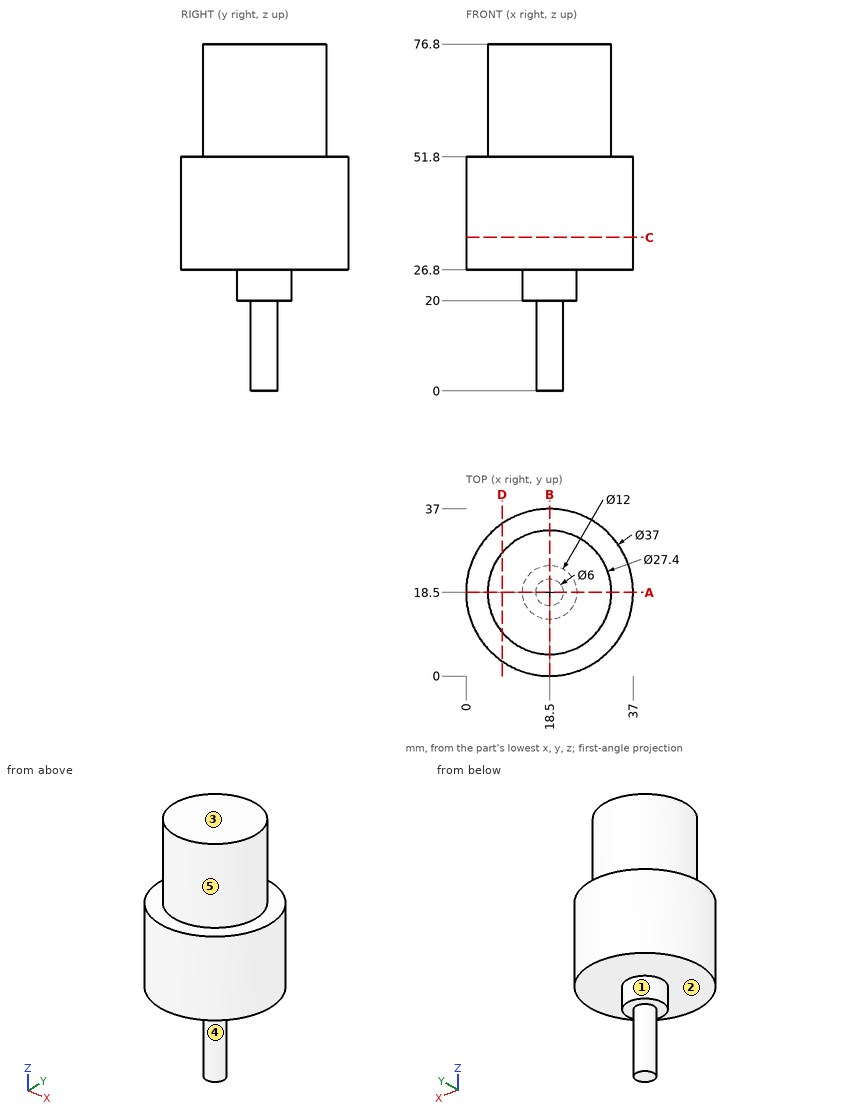
Source: three-view drawing plus pictorial views. Frame: mm from the lowest corner of the part. A direction names the side the tool comes from. Coordinates: 2 decimals unless noted, no trailing zeros. Write each loop counter-clockwise with the first axis right and the second up, starting at its lowest first coordinate (ties: lowest second). Pieces come first, ordered by that corner, then holes. Notation, with made-up numbers: (-3, 73.5) - (41, 73.5) arc R35 cw to (41, 108.5) - close; hole circle Ø6 at (-32, 30). An arc over 180 degrees is marked (long way). Answer as a JSON object with one key per item and string values.
Q1. Material intervals for line 1 (Z direction, x = 20, y = 25); line 2 (Z direction, x = 2, y = 15); line 3 (X direction, y = 29, z = 48), sorted ascending. Write a range as [from, to].
Ans:
{"line 1": "z = [26.8, 76.8]", "line 2": "z = [26.8, 51.8]", "line 3": "x = [3.27, 33.73]"}
Q2. Section query D-D, the plane x = 8. Output: boundary loops of the cut face in (y, z).
Ans:
{"outline": "(3.27, 26.8) - (33.73, 26.8) - (33.73, 51.8) - (27.3, 51.8) - (27.3, 76.8) - (9.7, 76.8) - (9.7, 51.8) - (3.27, 51.8) - close"}
Q3. First-contact query: pin 1 Ø12 at (x, z) = (26, 46.5) entering from +Y; pin 2 Ø6 at (x, z) = (21, 61.5) entering from +Y; pin 3 Ø12 at (y, z) = (17.5, 44.5) entering from -X; pin 4 Ø1.5 at (y, z) = (13, 46.5) entering from +X. Flat tips, straight axial feed; report the tip coordinate or a pass-through.
Ans:
{"pin 1": "stops at y = 36.94", "pin 2": "stops at y = 32.2", "pin 3": "stops at x = 0", "pin 4": "stops at x = 36.38"}
Q4. Set-up query: the marked faces 3, 4 and 5. Return all of +Z, -Z, +X, -X, +Y, -Y with unobstructed straight access to the full face (end or side cutting, diameter ignored); none if empty.
Ans:
{"face 3": "+Z, +X, -X, +Y, -Y", "face 4": "-Z", "face 5": "+Z"}
Q5. Section query A-A, the plane y = 18.5. Output: boundary loops of the cut face in (x, z).
Ans:
{"outline": "(0, 26.8) - (12.5, 26.8) - (12.5, 20) - (15.5, 20) - (15.5, 0) - (21.5, 0) - (21.5, 20) - (24.5, 20) - (24.5, 26.8) - (37, 26.8) - (37, 51.8) - (32.2, 51.8) - (32.2, 76.8) - (4.8, 76.8) - (4.8, 51.8) - (0, 51.8) - close"}
Q6. Section query C-C, the plane z = 34. Output: boundary loops of the cut face in (x, y), plus the area to 3 significant figures.
Ans:
{"outline": "circle Ø37 at (18.5, 18.5)", "area": "1,080 mm2"}
Q7. Draft query along X for the marked faces 1 and 2. Return one class per face: released by +X, released by -X, zero draft, split by the parting line, or undercut.
Ans:
{"face 1": "split by the parting line", "face 2": "zero draft"}
